Read the model definition and answer for the solid it produces. Units are mm, in the model's axes. Face numbers are marked on the shaded views. A direction names the side the tool comes from. Give positions to 0.01 mm unless a question says otherwise; leave off trailing zeros. Loops run counter-clockwise (first coordinate to the right, second up) from the corner with the lowest first, then second, coordinate; pieces in that order, holes last. Notation, with made-up numbers: (87.5, -29) - (128.5, -29) arc R4 ccw to (128.5, -22) - close; hole circle Ø11 at (-28, 42.5). An arc over 180 degrees is marked (long way). Write each question's results on one line, items separated by ' | '. Start each with the question number.
Q1. The part is cut by section C-C, the plane x = 0.4. Write down the section's boundary in (y, z).
Q2. For the marked faces 4, 5 and 6, determine the directions among +Z, -Z, +X, -X, +Y, -Y from which every point of the face is accessible in a straight line to the end or side of a thin tool.
Q3. Given pin 1 (2 mm diameter, centred on x = 1.5, z = 2, fed in from -Y); pin 2 (1.7 mm diameter, centred on x = 0.5, z = 3, fed in from -Y), each flat-ended and moving along its own axis, determine where each tip first touches the part or whether it passes through.
Q4. Find the intervals of material crossed by line 1 (Z direction, x = 0, y = 0.95); line 2 (Z direction, x = -1.25, y = 0.2); line 3 (X direction, y = 1.2, z = -1), in increasing order. Write a range as from..to.
Q5. Determine the mould class of the marked faces 1, 2 and 3 for opening direction Z: +Z half, -Z half, draft (parallel to the pull), parting line (faces both ways), or undercut.
Q6. The part is cut by section D-D, the plane y = 3.65. Write down the section's boundary in (x, z), plus the area to 3 significant figures.
Q7. The part is cut by section B-B, the plane z = 1.25. Write down the section's boundary in (x, y), plus the area to 3 significant figures.
Q8. The part is cut by section A-A, the plane y = 0.4. Write down the section's boundary in (x, z), plus the area to 3 significant figures.
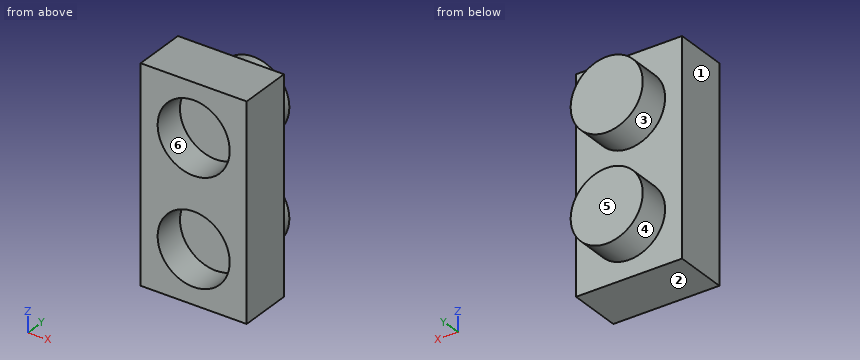
Autodesk Inventor part; units mm, degrees
ref_plane "YZ Plane" through (0, 0, 0) normal (1, 0, 0) x (0, 1, 0)
ref_plane "XZ Plane" through (0, 0, 0) normal (0, 1, 0) x (-1, 0, 0)
ref_plane "XY Plane" through (0, 0, 0) normal (0, 0, 1) x (1, 0, 0)
sketch "草圖1" plane through (0, 0, 0) normal (0, 1, 0) x (-1, 0, 0)
  line L0 (2.5, 5) -> (-2.5, 5)
  line L1 (-2.5, 5) -> (-2.5, -5)
  line L2 (-2.5, -5) -> (2.5, -5)
  line L3 (2.5, -5) -> (2.5, 5)
  circle A0 centre (0, 2.5) radius 1.7
  line L4 (2.5, 0) -> (-2.5, 0) construction
  circle A1 centre (0, -2.5) radius 1.7
  point P0 (0, 0)
  point P1 (0, -5)
  dimension "d0" = 5
  dimension "d1" = 10
  dimension "d2" = 3.4
  dimension "d3" = 2.5
  dimension "d4" = 2.5
extrude "擠出1" add sketch "草圖1" along normal blind 2.5 contours L3 L2 L1 L0 | A0 | A1
extrude "擠出2" cut sketch "草圖1" along normal blind 1.5 contours A0 | A1
sketch "草圖2" plane through (0, 2.5, 0) normal (0, 1, 0) x (1, 0, 0)
  circle A0 centre (0, -2.5) radius 1.7
  circle A1 centre (0, 2.5) radius 1.7
  point P0 (0, 0)
extrude "擠出3" add sketch "草圖2" along normal blind 1.5
properties part number "110033226_ipt_06_磚塊樺木(2x1)"
Check sheet entries:
1) outline: (0, -5) - (2.5, -5) - (2.5, -4.15) - (4, -4.15) - (4, -0.85) - (2.5, -0.85) - (2.5, 0.85) - (4, 0.85) - (4, 4.15) - (2.5, 4.15) - (2.5, 5) - (0, 5) - (0, 4.15) - (1.5, 4.15) - (1.5, 0.85) - (0, 0.85) - (0, -0.85) - (1.5, -0.85) - (1.5, -4.15) - (0, -4.15) - close
2) face 4: +Y | face 5: +Z, -Z, +X, -X, +Y | face 6: -Y
3) pin 1: stops at y = 0 | pin 2: stops at y = 1.5
4) line 1: z = -5..-4.2, -0.8..0.8, 4.2..5 | line 2: z = -5..-3.65, -1.35..1.35, 3.65..5 | line 3: x = -2.5..-0.8, 0.8..2.5
5) face 1: draft | face 2: -Z half | face 3: undercut
6) outline: circle Ø3.4 at (0, -2.5); circle Ø3.4 at (0, 2.5) | area: 18.2 mm^2
7) outline: (-2.5, 0) - (-1.15, 0) - (-1.15, 1.5) - (1.15, 1.5) - (1.15, 0) - (2.5, 0) - (2.5, 2.5) - (1.15, 2.5) - (1.15, 4) - (-1.15, 4) - (-1.15, 2.5) - (-2.5, 2.5) - close | area: 12.5 mm^2
8) outline: (-2.5, -5) - (2.5, -5) - (2.5, 5) - (-2.5, 5) - close; hole circle Ø3.4 at (0, -2.5); hole circle Ø3.4 at (0, 2.5) | area: 31.8 mm^2
